Check sheet for the modelled part. Datum: model origin and axes. Units: mm. A direction names the side the tool comes from. Round coordinates to 2 decimals unless told otherwise and drop trailing zeros. Order: outer loops, then holes, each group sorted by start corner. A loop starts at its lowest first (then second) coordinate and runs counter-clockwise, first axis right, second up. Notation, with made-up numbers: (40.25, 17.5) -> (65.25, 17.5) arc R18 cw to (65.25, 37.5) -> close; hole circle Ø10 at (55, 35). An arc over 180 degrees is marked (long way). Use CSV: the item, a comma, the result in double quotes.
Autodesk Inventor part; units mm, degrees
ref_plane "YZ Plane" through (0, 0, 0) normal (1, 0, 0) x (0, 1, 0)
ref_plane "XZ Plane" through (0, 0, 0) normal (0, 1, 0) x (-1, 0, 0)
ref_plane "XY Plane" through (0, 0, 0) normal (0, 0, 1) x (1, 0, 0)
sketch "Sketch1" plane through (0, 0, 0) normal (0, 0, 1) x (1, 0, 0)
  line L0 (0, 4) -> (0, 0)
  line L1 (0, 0) -> (125, 0)
  line L2 (0, 4) -> (57, 23.5)
  line L3 (103, 14.5) -> (103, 8)
  line L4 (103, 8) -> (73, 8)
  line L5 (73, 8) -> (73, 14.5)
  line L6 (125, 14.5) -> (121, 14.5)
  line L7 (121, 14.5) -> (121, 8)
  line L8 (121, 8) -> (125, 8)
  line L9 (125, 0) -> (125, 8)
  line L10 (125, 14.5) -> (125, 23.5)
  line L11 (81, 23.5) -> (81, 14.5)
  line L12 (92, 14.5) -> (92, 23.5)
  line L13 (73, 14.5) -> (81, 14.5)
  line L14 (92, 14.5) -> (103, 14.5)
  line L15 (81, 14.5) -> (92, 14.5) construction
  circle A0 centre (86.5, 19.599) radius 7.5 construction
  circle A1 centre (86.5, 19.599) radius 4 construction
  line L16 (113.5, 21.9084) -> (113.5, 17.2896)
  line L17 (113.5, 17.2896) -> (109.5, 14.9802)
  line L18 (109.5, 14.9802) -> (105.5, 17.2896)
  line L19 (105.5, 17.2896) -> (105.5, 21.9084)
  line L20 (105.5, 21.9084) -> (109.5, 24.2178)
  line L21 (109.5, 24.2178) -> (113.5, 21.9084)
  circle A2 centre (109.5, 19.599) radius 2.5 construction
  line L22 (103.5, 23.5) -> (103.5, 29.5)
  line L23 (105.5, 31.5) -> (113.5, 31.5)
  line L24 (115.5, 29.5) -> (115.5, 23.5)
  arc A3 (105.5, 31.5) -> (103.5, 29.5) centre (105.5, 29.5) ccw
  arc A4 (115.5, 29.5) -> (113.5, 31.5) centre (113.5, 29.5) ccw
  line L25 (125, 23.5) -> (115.5, 23.5)
  line L26 (103.5, 23.5) -> (92, 23.5)
  circle A5 centre (99.5, 19) radius 4.5 construction
  circle A6 centre (119.5, 19) radius 4.5 construction
  circle A7 centre (99.5, 19) radius 2.25
  circle A8 centre (119.5, 19) radius 2.25
  line L27 (67, 23.5) -> (67, 29.5)
  line L28 (69, 31.5) -> (73, 31.5)
  line L29 (75, 29.5) -> (75, 23.5)
  arc A9 (69, 31.5) -> (67, 29.5) centre (69, 29.5) ccw
  arc A10 (75, 29.5) -> (73, 31.5) centre (73, 29.5) ccw
  line L30 (81, 23.5) -> (75, 23.5)
  line L31 (67, 23.5) -> (57, 23.5)
  point P0 (81, 14.5)
  point P1 (92, 14.5)
  point P2 (86.5, 14.5)
  point P3 (125, 19)
  point P4 (109.5, 31.5)
  dimension "d0" = 8
  dimension "d2" = 6.5
  dimension "d3" = 4
  dimension "d4" = 15
  dimension "d5" = 8
  dimension "d6" = 9
  dimension "d7" = 11
  dimension "d8" = 11
  dimension "d9" = 8
  dimension "d10" = 5
  dimension "d11" = 2
  dimension "d12" = 12
  dimension "d13" = 9
  dimension "d14" = 9
  dimension "d15" = 10
  dimension "d16" = 10
  dimension "d17" = 4.5
  dimension "d18" = 4.5
  dimension "d19" = 13
  dimension "d20" = 5.5
  dimension "d21" = 18
  dimension "d22" = 2
  dimension "d23" = 8
  dimension "d24" = 6
  dimension "d25" = 10
  dimension "d27" = 30
  dimension "d28" = 4
  dimension "d30" = 8
  dimension "d31" = 125
extrude "Extrusion1" add sketch "Sketch1" along normal blind 6.5
sketch "Sketch2" plane through (0, 0, 6.5) normal (0, 0, 1) x (1, 0, 0)
  line L0 (0, 4) -> (0, 0)
  line L1 (0, 0) -> (125, 0)
  line L2 (6, 0) -> (14, 0)
  line L3 (14, 0) -> (14, -4.5)
  line L4 (12, -6.5) -> (8, -6.5)
  line L5 (6, -4.5) -> (6, 0)
  line L6 (57, 0) -> (65, 0)
  line L7 (65, 0) -> (65, -4.5)
  line L8 (63, -6.5) -> (59, -6.5)
  line L9 (57, -4.5) -> (57, 0)
  line L10 (85, 0) -> (93, 0)
  line L11 (93, 0) -> (93, -4.5)
  line L12 (91, -6.5) -> (87, -6.5)
  line L13 (85, -4.5) -> (85, 0)
  line L14 (113, 0) -> (121, 0)
  line L15 (121, 0) -> (121, -4.5)
  line L16 (119, -6.5) -> (115, -6.5)
  line L17 (113, -4.5) -> (113, 0)
  arc A0 (6, -4.5) -> (8, -6.5) centre (8, -4.5) ccw
  arc A1 (12, -6.5) -> (14, -4.5) centre (12, -4.5) ccw
  arc A2 (57, -4.5) -> (59, -6.5) centre (59, -4.5) ccw
  arc A3 (63, -6.5) -> (65, -4.5) centre (63, -4.5) ccw
  arc A4 (85, -4.5) -> (87, -6.5) centre (87, -4.5) ccw
  arc A5 (91, -6.5) -> (93, -4.5) centre (91, -4.5) ccw
  arc A6 (113, -4.5) -> (115, -6.5) centre (115, -4.5) ccw
  arc A7 (119, -6.5) -> (121, -4.5) centre (119, -4.5) ccw
  dimension "d34" = 2
  dimension "d35" = 8
  dimension "d36" = 8
  dimension "d37" = 8
  dimension "d38" = 8
  dimension "d39" = 6.5
  dimension "d40" = 6
  dimension "d41" = 43
  dimension "d42" = 20
  dimension "d43" = 20
extrude "Extrusion2" add sketch "Sketch2" against normal blind 6.5
sketch "Sketch3" plane through (0, 0, 6.5) normal (0, 0, 1) x (1, 0, 0)
  line L0 (0, 4) -> (0, 0)
  line L1 (14, 0) -> (57, 0)
  circle A0 centre (28.2, 6) radius 2.25
  circle A1 centre (28.2, 6) radius 4.5 construction
  dimension "d46" = 4.5
  dimension "d47" = 6
  dimension "d48" = 28.2
  dimension "d51" = 9
extrude "Extrusion3" cut sketch "Sketch3" against normal through all
properties part number "x_motor_wall_upper"
Q1. Sectioned sample at B-B, the plane y = 26. Enter the section's corners in (x, z).
Result sheet:
outline,"(67, 0) -> (75, 0) -> (75, 6.5) -> (67, 6.5) -> close; (103.5, 0) -> (115.5, 0) -> (115.5, 6.5) -> (103.5, 6.5) -> close"
Q2. Sectioned sample at C-C, the plane y = 19. Enter the section's corners in (x, z), then the cut area to 4 significant figures.
Result sheet:
outline,"(43.85, 0) -> (81, 0) -> (81, 6.5) -> (43.85, 6.5) -> close; (92, 0) -> (97.25, 0) -> (97.25, 6.5) -> (92, 6.5) -> close; (101.75, 0) -> (105.5, 0) -> (105.5, 6.5) -> (101.75, 6.5) -> close; (113.5, 0) -> (117.25, 0) -> (117.25, 6.5) -> (113.5, 6.5) -> close; (121.75, 0) -> (125, 0) -> (125, 6.5) -> (121.75, 6.5) -> close"
area,"345.5 mm^2"
Q3. Sectioned sample at D-D, the plane z = 5. State how many separate pieces and enclosed holes the cut face has, then the cut area to 3 significant figures.
Result sheet:
separate pieces,"1"
enclosed holes,"4"
area,"2,320 mm^2"
Q4. Scan lines: L1, parallel to X at y = -4, z = 4.5; L2, parallel to X at y = 24, z = 0.75; L3, parallel to Y at x = 59, z = 0.75. Record each from-to range of solid material in increasing order.
Result sheet:
L1,"x = 6 to 14, 57 to 65, 85 to 93, 113 to 121"
L2,"x = 67 to 75, 103.5 to 109.12, 109.88 to 115.5"
L3,"y = -6.5 to 23.5"
Q5. Go/stop test with flat-tipped pins: pin 1 (3 mm diameter, centred on x = 88, z = 4, fed in from +Y); pin 2 (2 mm diameter, centred on x = 40.5, z = 4, fed in from -Y); pin 3 (1 mm diameter, centred on x = 111, y = 21, fed in from +Z); pin 4 (1.2 mm diameter, centred on x = 123, z = 5, fed in from +Y). Record where each tip stops, or that it passes through.
Result sheet:
pin 1,"stops at y = 8"
pin 2,"stops at y = 0"
pin 3,"passes through"
pin 4,"stops at y = 23.5"
Q6. Sectioned sample at A-A, the plane x = 76.5. Enter the section's corners in (y, z).
Result sheet:
outline,"(0, 0) -> (8, 0) -> (8, 6.5) -> (0, 6.5) -> close; (14.5, 0) -> (23.5, 0) -> (23.5, 6.5) -> (14.5, 6.5) -> close"
Q7. Access from +Z, -Z, +X, -X, +Y, -Y to the whole of each face (thin tool, end or side, straight path). Record for faces 4 (the face through (92, 19, 3)), 5 (the face through (62, 23.5, 3)), 6 (the face through (85, -2, 3)).
Result sheet:
face 4,"+Z, -Z, +Y"
face 5,"+Z, -Z, -X, +Y"
face 6,"+Z, -Z, -Y"
Q8. Mould release check, pull along X, two halves, no side actions. Record for faces 1 (the face through (120.4, -5.93, 3.3)), 2 (the face through (117, -6.5, 3)), 3 (the face through (73, 11, 3)): pulls with the +X half, pulls with the -X half, needs draft (parallel to the pull), parting line crosses it, or undercut.
Result sheet:
face 1,"pulls with the +X half"
face 2,"needs draft"
face 3,"undercut"
